Verification items for the finished model (mm, model axes). Face numbers are marked on the shaded views. A direction names the side the tool comes from. Round coordinates to 2 decimals unless told otherwise and drop trailing zeros. Order: outer loops, then holes, each group sorted by start corner. A loop starts at its lowest first (then second) coordinate and runs counter-clockwise, first axis right, second up. Notation, with made-up numbers: (-11, 11.5) -> (-5, 11.5) arc R21 ccw to (-5, 19.5) -> close; hole circle Ø2 at (51, 42). An arc over 180 degrees is marked (long way). Put each result on its own line as item: value.
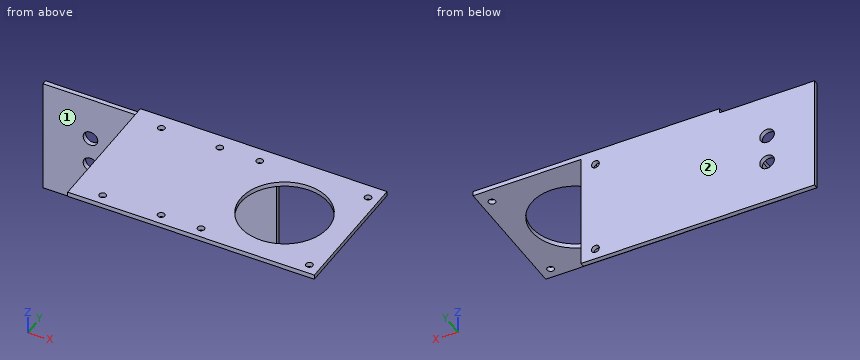
```python
from build123d import *

# Parameters (mm, degrees)
SKETCH1_W           = 107.2
SKETCH1_H           = 58.4
SKETCH1_R           = 1.5
SKETCH1_R_2         = 19.05
BOSS_EXTRUDE1_DEPTH = 2
BOSS_EXTRUDE2_DEPTH = 50.8
SKETCH3_R           = 1.7
SKETCH3_R_2         = 3.175
CUT_EXTRUDE1_DEPTH  = 134.004661572


with BuildPart() as part:
    # Sketch1 → Boss-Extrude1 (new body)
    with BuildSketch(Plane.XY):
        with Locations((53.6, 29.2)):
            Rectangle(SKETCH1_W, SKETCH1_H)
        with Locations((102.55, 51.75)):
            Circle(SKETCH1_R, mode=Mode.SUBTRACT)
        with Locations((102.55, 4.65)):
            Circle(SKETCH1_R, mode=Mode.SUBTRACT)
        with Locations((55.45, 4.65)):
            Circle(SKETCH1_R, mode=Mode.SUBTRACT)
        with Locations((55.45, 51.75)):
            Circle(SKETCH1_R, mode=Mode.SUBTRACT)
        with Locations((12.7, 51.75)):
            Circle(SKETCH1_R, mode=Mode.SUBTRACT)
        with Locations((38.1, 51.75)):
            Circle(SKETCH1_R, mode=Mode.SUBTRACT)
        with Locations((12.7, 4.65)):
            Circle(SKETCH1_R, mode=Mode.SUBTRACT)
        with Locations((38.1, 4.65)):
            Circle(SKETCH1_R, mode=Mode.SUBTRACT)
        with Locations((79, 28.2)):
            Circle(SKETCH1_R_2, mode=Mode.SUBTRACT)
    extrude(amount=-BOSS_EXTRUDE1_DEPTH)

    # Sketch2 → Boss-Extrude2 (add)
    with BuildSketch(Plane(origin=(0, 0, -2), x_dir=(-1, 0, 0), z_dir=(0, 0, -1))):
        Polygon((0, 56.4), (41.275, 56.4), (41.275, 58.4), (0, 58.4), (-60.325, 58.4), (-60.325, 56.4), align=None)
    extrude(amount=BOSS_EXTRUDE2_DEPTH)

    # Sketch3 → Cut-Extrude1 (cut, through all)
    with BuildSketch(Plane(origin=(0, 58.4, 0), x_dir=(1, 0, 0), z_dir=(0, 1, 0))):
        with Locations(Location((53.975, 48.0375, 0), (0, 0, 180))):
            Circle(SKETCH3_R)
        with Locations(Location((53.975, 6.7625, 0), (0, 0, 180))):
            Circle(SKETCH3_R)
        with Locations(Location((-20.6375, 33.75, 0), (0, 0, 180))):
            Circle(SKETCH3_R_2)
        with Locations(Location((-20.6375, 21.05, 0), (0, 0, 180))):
            Circle(SKETCH3_R_2)
    extrude(amount=-CUT_EXTRUDE1_DEPTH, mode=Mode.SUBTRACT)


solid = part.part
```
Item 1: Sectioned sample at C-C, the plane y = 4.65. Record the boundary of the cut face in (x, z), then the cut area to 3 significant figures.
Geometry check:
outline: (0, -2) -> (11.2, -2) -> (11.2, 0) -> (0, 0) -> close; (14.2, -2) -> (36.6, -2) -> (36.6, 0) -> (14.2, 0) -> close; (39.6, -2) -> (53.95, -2) -> (53.95, 0) -> (39.6, 0) -> close; (56.95, -2) -> (101.05, -2) -> (101.05, 0) -> (56.95, 0) -> close; (104.05, -2) -> (107.2, -2) -> (107.2, 0) -> (104.05, 0) -> close
area: 190 mm2
Item 2: Sectioned sample at A-A, the plane x = 12.7. Record the boundary of the cut face in (y, z), then the cut area to 3 significant figures.
Geometry check:
outline: (0, -2) -> (3.15, -2) -> (3.15, 0) -> (0, 0) -> close; (6.15, -2) -> (50.25, -2) -> (50.25, 0) -> (6.15, 0) -> close; (53.25, -2) -> (56.4, -2) -> (56.4, -52.8) -> (58.4, -52.8) -> (58.4, 0) -> (53.25, 0) -> close
area: 206 mm2
Item 3: Tool access check on the marked faces 1 and 2. Record the directions out of +Z, -Z, +X, -X, +Y, -Y that give a thin tool (end or side, any length) a straight path to the whole face; none if there is none.
Geometry check:
face 1: -Z, +X, -X, -Y
face 2: +Z, -Z, +X, -X, +Y
Item 4: Depth check by flat-ended pin: pin 1 Ø3 at (x, z) = (57.5, -10) entering from -Y; pin 2 Ø2.5 at (x, y) = (12.7, 4.65) entering from +Z; pin 3 Ø4 at (x, y) = (67, 43.5) entering from -Z; pin 4 Ø0.6 at (x, y) = (-17.5, 57.5) entering from +Z. Enter the tip coordinate at first touch or a pass-through.
Geometry check:
pin 1: y = 56.4
pin 2: through
pin 3: z = -2
pin 4: z = -2
Item 5: Sectioned sample at B-B, the plane z = -33.75. Record the boundary of the cut face in (x, y) (1 decimal), then the cut area to 4 significant figures.
Geometry check:
outline: (-41.3, 56.4) -> (-23.8, 56.4) -> (-23.8, 58.4) -> (-41.3, 58.4) -> close; (-17.5, 56.4) -> (60.3, 56.4) -> (60.3, 58.4) -> (-17.5, 58.4) -> close
area: 190.5 mm2
Item 6: Material ranges on line 1 along Y through (x, z) = (102.55, -0.7); line 2 along Z through (x, y) = (95.5, 5); line 3 along Y through (x, z) = (-35, -35.5), recorded low to high.
Geometry check:
line 1: 0 to 3.15, 6.15 to 50.25, 53.25 to 58.4
line 2: -2 to 0
line 3: 56.4 to 58.4
Item 7: Sectioned sample at D-D, the plane y = 22.5. Record the boundary of the cut face in (x, z), then the cut area to 3 significant figures.
Geometry check:
outline: (0, -2) -> (60.82, -2) -> (60.82, 0) -> (0, 0) -> close; (97.18, -2) -> (107.2, -2) -> (107.2, 0) -> (97.18, 0) -> close
area: 142 mm2
